Can you work these out from the model? Positions are in its coordinate system, mm. A direction names the side the tool comes from. Round coordinates to 2 decimals unless told otherwise and drop trailing zeros. Write each loop counter-clockwise with the first axis right and the second up, starting at its lowest first coordinate (ties: lowest second). Pieces come first, ordered by that corner, then holes. Notation, with made-up numbers: M -35.75,35 L -13.75,35 A25 ccw -13.75,57 Z; hole C -14,-33 d9. An arc over 180 degrees is marked long. Answer as a JSON object with one key per item and string values. Group by question number.
1) Suppose I cut it at A-A, the plane x = 0. Write out the boundary of the cut face in (y, z).
2) Suppose I cut it at C-C, the plane z = 7. Write out the boundary of the cut face in (x, y).
3) Please list where these lines run through material, in increasing order: L1, parallel to Z at x = -5.5, y = 2.5; L2, parallel to Y at x = 0, z = 51.5; L3, parallel to Y at x = 3.25, z = 95.5. Write a range as [from, to].
4) On a 3-axis mill with a long thin cutter (end or side, diameter ignored), from which of +Z, -Z, +X, -X, +Y, -Y can I reach the whole of each face in a straight line? I mean faces 1 (the flat face through (0, 0, 0)), 2 (the cylindrical face through (-6, 0, 50)), 3 (the cylindrical face through (6.466, -2.681, 43.479)), 4 (the cylindrical face through (-6, 0, 21)), 5 (the flat face through (6, 2, 58)). Say none if no direction works.
5) I'm going to push flat-ended pins straight in: pin 1 Ø1.5 at (y, z) = (3, 18.5) entering from -X; pin 2 Ø1 at (y, z) = (-4.5, 44.5) entering from -X; pin 3 Ø1 at (y, z) = (-2.5, 25) entering from +X. Where does each tip first touch, or does it pass through?
6) If we mould it in two halves opening along Z, with no side actions, what happens to faces 6 (the cylindrical face through (-6, 0, 79)), 7 (the flat face through (0, 0, 100)), 8 (the flat face through (6, 2, 55))? For each: +Z half, -Z half, draft (parallel to the pull), parting line (faces both ways), or undercut.
from build123d import *

# Parameters (mm, degrees)
SKETCH1_R           = 6
BOSS_EXTRUDE1_DEPTH = 42
SKETCH2_R           = 7
BOSS_EXTRUDE2_DEPTH = 3
SKETCH3_R           = 6
BOSS_EXTRUDE3_DEPTH = 10
SKETCH4_R           = 7
BOSS_EXTRUDE4_DEPTH = 3
SKETCH5_R           = 6
BOSS_EXTRUDE5_DEPTH = 42


with BuildPart() as part:
    # Sketch1 → Boss-Extrude1 (new body)
    with BuildSketch(Plane.XY):
        Circle(SKETCH1_R)
    extrude(amount=BOSS_EXTRUDE1_DEPTH)

    # Sketch2 → Boss-Extrude2 (add)
    with BuildSketch(Plane.XY.offset(42)):
        Circle(SKETCH2_R)
    extrude(amount=BOSS_EXTRUDE2_DEPTH)

    # Sketch3 → Boss-Extrude3 (add)
    with BuildSketch(Plane.XY.offset(45)):
        Circle(SKETCH3_R)
    extrude(amount=BOSS_EXTRUDE3_DEPTH)

    # Sketch4 → Boss-Extrude4 (add)
    with BuildSketch(Plane.XY.offset(55)):
        Circle(SKETCH4_R)
    extrude(amount=BOSS_EXTRUDE4_DEPTH)

    # Sketch5 → Boss-Extrude5 (add)
    with BuildSketch(Plane.XY.offset(58)):
        Circle(SKETCH5_R)
    extrude(amount=BOSS_EXTRUDE5_DEPTH)


solid = part.part
Results:
{
 "1": {"outline": "M -7,42 L -6,42 L -6,0 L 6,0 L 6,42 L 7,42 L 7,45 L 6,45 L 6,55 L 7,55 L 7,58 L 6,58 L 6,100 L -6,100 L -6,58 L -7,58 L -7,55 L -6,55 L -6,45 L -7,45 Z"},
 "2": {"outline": "C 0,0 d12"},
 "3": {"L1": "[42, 45], [55, 58]", "L2": "[-6, 6]", "L3": "[-5.04, 5.04]"},
 "4": {"face 1": "-Z, +X, -X, +Y, -Y", "face 2": "none", "face 3": "+Z, -Z", "face 4": "-Z", "face 5": "+Z"},
 "5": {"pin 1": "x = -5.56", "pin 2": "x = -5.74", "pin 3": "x = 5.66"},
 "6": {"face 6": "draft", "face 7": "+Z half", "face 8": "undercut"}
}
